from build123d import *

# Parameters (mm, degrees)
CROQUIS1_R              = 11
CROQUIS1_R_2            = 2
CROQUIS1_W              = 30
CROQUIS1_H              = 3
SALIENTE_EXTRUIR1_DEPTH = 3
CROQUIS2_R              = 13
CROQUIS2_R_2            = 11
SALIENTE_EXTRUIR2_DEPTH = 4
CROQUIS3_R              = 13
CROQUIS3_R_2            = 9
SALIENTE_EXTRUIR3_DEPTH = 2
CHAFL_N1_SIZE           = 2
CHAFL_N2_SIZE           = 10
CROQUIS6_W              = 9.75
CROQUIS6_H              = 19.6
CROQUIS6_R              = 2.25
CORTAR_EXTRUIR2_DEPTH   = 1.5


with BuildPart() as part:
    # Croquis1 → Saliente-Extruir1 (new body)
    with BuildSketch(Plane(origin=(0, 0, 0), x_dir=(1, 0, 0), z_dir=(0, 1, 0))):
        Polygon((-67.5, -20), (67.5, -20), (67.5, -9.8), (77.25, -9.8), (77.25, 9.8), (67.5, 9.8), (67.5, 20), (-67.5, 20), align=None)
        with Locations(Location((-48.5, 0, 0), (0, 0, 270))):
            Circle(CROQUIS1_R, mode=Mode.SUBTRACT)
        with Locations(Location((-23.5, 0, 0), (0, 0, 270))):
            Circle(CROQUIS1_R_2, mode=Mode.SUBTRACT)
        with Locations(Location((-8.5, 0, 0), (0, 0, 270))):
            Circle(CROQUIS1_R_2, mode=Mode.SUBTRACT)
        with Locations(Location((52.5, 0, 0), (0, 0, 270))):
            Circle(CROQUIS1_R_2, mode=Mode.SUBTRACT)
        with Locations((27.5, 11)):
            Rectangle(CROQUIS1_W, CROQUIS1_H, mode=Mode.SUBTRACT)
        with Locations((27.5, -11)):
            Rectangle(CROQUIS1_W, CROQUIS1_H, mode=Mode.SUBTRACT)
    extrude(amount=SALIENTE_EXTRUIR1_DEPTH)

    # Croquis2 → Saliente-Extruir2 (add)
    with BuildSketch(Plane(origin=(0, 3, 0), x_dir=(1, 0, 0), z_dir=(0, 1, 0))):
        with Locations(Location((-48.5, 0, 0), (0, 0, 90))):
            Circle(CROQUIS2_R)
        with Locations(Location((-48.5, 0, 0), (0, 0, 270))):
            Circle(CROQUIS2_R_2, mode=Mode.SUBTRACT)
    extrude(amount=SALIENTE_EXTRUIR2_DEPTH)

    # Croquis3 → Saliente-Extruir3 (add)
    with BuildSketch(Plane(origin=(0, 7, 0), x_dir=(1, 0, 0), z_dir=(0, 1, 0))):
        with Locations(Location((-48.5, 0, 0), (0, 0, 90))):
            Circle(CROQUIS3_R)
        with Locations(Location((-48.5, 0, 0), (0, 0, 270))):
            Circle(CROQUIS3_R_2, mode=Mode.SUBTRACT)
    extrude(amount=SALIENTE_EXTRUIR3_DEPTH)

    # Chaflán1
    chafl_n1_edges = [part.edges().sort_by_distance(p)[0] for p in [
        (-48.5, 9, 13),
    ]]
    chamfer(chafl_n1_edges, length=CHAFL_N1_SIZE)

    # Chaflán2
    chafl_n2_edges = [part.edges().sort_by_distance(p)[0] for p in [
        (-67.5, 1.5, 20),
        (-67.5, 1.5, -20),
    ]]
    chamfer(chafl_n2_edges, length=CHAFL_N2_SIZE)

    # Croquis6 → Cortar-Extruir2 (cut)
    with BuildSketch(Plane(origin=(0, 3, 0), x_dir=(1, 0, 0), z_dir=(0, 1, 0))):
        with Locations((72.375, 0)):
            Rectangle(CROQUIS6_W, CROQUIS6_H)
        with Locations(Location((72.375, 0, 0), (0, 0, 270))):
            Circle(CROQUIS6_R, mode=Mode.SUBTRACT)
    extrude(amount=-CORTAR_EXTRUIR2_DEPTH, mode=Mode.SUBTRACT)


solid = part.part
Source: CAD feature listing. Evaluate the final solid. Frame: model axes, mm. A direction names the side the tool comes from. Give positions to 0.01 mm unless a question says otherwise; leave off trailing zeros. Write each loop counter-clockwise with the first axis right and the second up, starting at its lowest first coordinate (ties: lowest second). Pieces come first, ordered by that corner, then holes. Notation, with made-up numbers: M 36,62 L 87,62 A29 cw 87,92 Z; hole C 2.5,34.5 d6. An arc over 180 degrees is marked long. Return JSON: item names as keys, results as strings. Group by question number.
1) Cut plane A-A, the plane x = 14. Output: boundary loops of the cut face in (y, z).
2) Cut plane C-C, the plane z = 0. Give the number of separate pieces and of enclosed holes in the cut face, then the cut area to 3 significant figures.
3) Set-up query: faces 1 (the face through (6, 1, -20)), 2 (the face through (27, 1, 9.5)), 3 (the face through (-61.39, 4.97, 1.69)), 4 (the face through (72, 3, 0)), 5 (the face through (-62.6, 1.5, 14.9)). Return all of +Z, -Z, +X, -X, +Y, -Y with unobstructed straight access to the full face (end or side cutting, diameter ignored); none if empty.
4) Cut plane B-B, the plane x = -48.5. Output: boundary loops of the cut face in (y, z), then the cut area to 3 significant figures.
5) Draft query along X for faces 6 (the face through (-67.5, 1, 0)), 7 (the face through (-40, 9, 4)), 8 (the face through (-40, 7, 4)). Return one class per face: released by +X, released by -X, zero draft, split by the parting line, or undercut.
6) Ray query, L1, parallel to X at y = 1.2, z = 0; L2, parallel to X at y = 1.85, z = 0 (3 decimals); L3, parallel to Z at x = 14, y = 0.75. Return the intervals inside material, ascending.
7) Cut plane D-D, the plane x = -23.5. Output: boundary loops of the cut face in (y, z), then the cut area to 3 significant figures.
8) First-contact query: pin 1 Ø1.6 at (x, y) = (70, 1) entering from +Z; pin 2 Ø1.2 at (x, y) = (71.5, 0.5) entering from -Z; pin 3 Ø20 at (x, z) = (-24, 8) entering from +Y. Flat tips, straight axial feed; report the tip coordinate or a pass-through.
Data:
{
 "1": {"outline": "M 0,-20 L 3,-20 L 3,-12.5 L 0,-12.5 Z; M 0,-9.5 L 3,-9.5 L 3,9.5 L 0,9.5 Z; M 0,12.5 L 3,12.5 L 3,20 L 0,20 Z"},
 "2": {"separate pieces": "5", "enclosed holes": "0", "area": "352 mm²"},
 "3": {"face 1": "-Z, +X, -X, +Y, -Y", "face 2": "+Y, -Y", "face 3": "+Y", "face 4": "+Z, -Z, +X, +Y", "face 5": "+Z, -X, +Y, -Y"},
 "4": {"outline": "M 0,-20 L 3,-20 L 3,-13 L 7,-13 L 9,-11 L 9,-9 L 7,-9 L 7,-11 L 0,-11 Z; M 0,11 L 7,11 L 7,9 L 9,9 L 9,11 L 7,13 L 3,13 L 3,20 L 0,20 Z", "area": "82.0 mm²"},
 "5": {"face 6": "released by -X", "face 7": "zero draft", "face 8": "undercut"},
 "6": {"L1": "x = -67.5 to -59.5, -37.5 to -25.5, -21.5 to -10.5, -6.5 to 50.5, 54.5 to 77.25", "L2": "x = -67.5 to -59.5, -37.5 to -25.5, -21.5 to -10.5, -6.5 to 50.5, 54.5 to 67.5, 70.125 to 74.625", "L3": "z = -20 to -12.5, -9.5 to 9.5, 12.5 to 20"},
 "7": {"outline": "M 0,-20 L 3,-20 L 3,-2 L 0,-2 Z; M 0,2 L 3,2 L 3,20 L 0,20 Z", "area": "108 mm²"},
 "8": {"pin 1": "stops at z = 9.8", "pin 2": "stops at z = -9.8", "pin 3": "stops at y = 3"}
}
